Design review of the part built by this model. Coordinates are the model's own, in mm. Give positions to 0.01 mm unless a question says otherwise; leave off trailing zeros. Loops run counter-clockwise (first coordinate to the right, second up) from the corner with the lowest first, then second, coordinate; pieces in that order, holes last. Notation, with made-up numbers: (43.25, 3) -> (87.25, 3) arc R23 cw to (87.25, 17) -> close; hole circle Ø7 at (38.5, 1). An arc over 180 degrees is marked (long way). Use CSV: the item, a comma, the result in double quotes. Start each with the question number.
Item 1: Clearance check with flat-ended pins moving along their axes: pin 1 (2.5 mm diameter, centred on y = 8.175, z = 65, fed in from -X); pin 2 (4.5 mm diameter, centred on y = 8.175, z = -65, fed in from +X) (3 decimals); pin 3 (4 mm diameter, centred on y = 55.35, z = 75, fed in from +X) (3 decimals). State where each tip first meets the part, or that it passes through.
Item 2: We need section B-B (z = -98). State the section outline as (x, y) points (3 decimals), plus the area to 3 significant figures.
Item 3: Wall thickness on line 1 along Z through (x, y) = (0.75, 55.35) (3 decimals); line 2 along Z through (x, y) = (0.55, 71) (3 decimals); line 3 along Y through (x, z) = (0.95, 65) (3 decimals): over which ranges is each line inside the solid? List them lowest first. Write a range as from..to.
Item 4: We need section A-A (y = 69.5). State the section outline as (x, z) points (3 decimals), plus the area to 3 significant figures.
from build123d import *

# Parameters (mm, degrees)
BOSS_EXTRUDE1_DEPTH                             = 3.175
CSK_FOR_M3_FLAT_HEAD_MACHINE_SCREW1_D           = 3.4
CSK_FOR_M3_FLAT_HEAD_MACHINE_SCREW1_CSINK_D     = 6.3
CSK_FOR_M3_FLAT_HEAD_MACHINE_SCREW1_CSINK_ANGLE = 90
CUT_EXTRUDE1_DEPTH                              = 4.175


with BuildPart() as part:
    # Sketch1 → Boss-Extrude1 (new body)
    with BuildSketch(Plane(origin=(0, 0, 0), x_dir=(0, 0, -1), z_dir=(1, 0, 0))):
        Polygon((103.175, 0), (103.175, 3.175), (103.175, 47.175), (103.175, 50.35), (103.175, 60.35), (103.175, 90.35), (-103.175, 90.35), (-103.175, 60.35), (-103.175, 50.35), (-103.175, 47.175), (-103.175, 3.175), (-103.175, 0), align=None)
    extrude(amount=BOSS_EXTRUDE1_DEPTH)

    # CSK for M3 Flat Head Machine Screw1 (through all)
    with Locations(Plane(origin=(3.175, 0, 0), x_dir=(0, 0, -1), z_dir=(1, 0, 0))):
        with Locations((-75, 8.175), (-65, 8.175), (-75, 55.35), (-65, 55.35), (-75, 85.35), (-65, 85.35)):
            csk_for_m3_flat_head_machine_screw1 = CounterSinkHole(CSK_FOR_M3_FLAT_HEAD_MACHINE_SCREW1_D / 2, CSK_FOR_M3_FLAT_HEAD_MACHINE_SCREW1_CSINK_D / 2, counter_sink_angle=CSK_FOR_M3_FLAT_HEAD_MACHINE_SCREW1_CSINK_ANGLE)

    # Mirror1: CSK for M3 Flat Head Machine Screw1 across plane
    add(csk_for_m3_flat_head_machine_screw1.mirror(Plane.XY), mode=Mode.SUBTRACT)

    # Sketch4 → Cut-Extrude1 (cut, through all)
    with BuildSketch(Plane(origin=(3.175, 0, 0), x_dir=(0, 0, -1), z_dir=(1, 0, 0))):
        with BuildLine():
            Line((-96, 73.35), (-96, 67.35))
            ThreePointArc((-96, 67.35), (-98, 65.35), (-100, 67.35))
            Line((-100, 67.35), (-100, 73.35))
            ThreePointArc((-100, 73.35), (-98, 75.35), (-96, 73.35))
        make_face()
        with BuildLine():
            Line((96, 73.35), (96, 67.35))
            ThreePointArc((96, 67.35), (98, 65.35), (100, 67.35))
            Line((100, 67.35), (100, 73.35))
            ThreePointArc((100, 73.35), (98, 75.35), (96, 73.35))
        make_face()
    extrude(amount=-CUT_EXTRUDE1_DEPTH, mode=Mode.SUBTRACT)


solid = part.part
Results found:
1,pin 1,"through"
1,pin 2,"x = 2.275"
1,pin 3,"x = 2.025"
2,outline,"(0, 0) -> (3.175, 0) -> (3.175, 65.35) -> (0, 65.35) -> close; (0, 75.35) -> (3.175, 75.35) -> (3.175, 90.35) -> (0, 90.35) -> close"
2,area,"255 mm²"
3,line 1,"-103.175..-76.7, -73.3..-66.7, -63.3..63.3, 66.7..73.3, 76.7..103.175"
3,line 2,"-103.175..-100, -96..96, 100..103.175"
3,line 3,"0..6.475, 9.875..53.65, 57.05..83.65, 87.05..90.35"
4,outline,"(0, -103.175) -> (3.175, -103.175) -> (3.175, -100) -> (0, -100) -> close; (0, -96) -> (3.175, -96) -> (3.175, 96) -> (0, 96) -> close; (0, 100) -> (3.175, 100) -> (3.175, 103.175) -> (0, 103.175) -> close"
4,area,"630 mm²"
